```python
from build123d import *

# Parameters (mm, degrees)
F0_R        = 3.175
F1_DEPTH    = 6.35
F2_R        = 3.175
F3_DEPTH    = 6.351
F5_DEPTH    = 6.351
F6_T1_DEPTH = 6.35
F7_R        = 1.5875


# Not quite as in the source:
# - a fillet or chamfer that OpenCascade refuses, or shapes differently, is made with other operations: its cross-section is extruded or revolved along the edge and cut away or added


with BuildPart() as f1:
    # F0 (on Front) → F1 (new body)
    with BuildSketch(Plane.XZ):
        with BuildLine():
            ThreePointArc((32.9955678842, -27.305), (40.1446075924, -23.1775), (40.1446075924, -14.9225))
            Line((40.1446075924, -14.9225), (7.1490397082, 42.2275))
            ThreePointArc((7.1490397082, 42.2275), (0, 46.355), (-7.1490397082, 42.2275))
            Line((-7.1490397082, 42.2275), (-40.1446075924, -14.9225))
            ThreePointArc((-40.1446075924, -14.9225), (-40.1446075924, -23.1775), (-32.9955678842, -27.305))
            Line((-32.9955678842, -27.305), (32.9955678842, -27.305))
        make_face()
        with Locations((-32.9955678842, -19.05)):
            Circle(F0_R, mode=Mode.SUBTRACT)
        with Locations((32.9955678842, -19.05)):
            Circle(F0_R, mode=Mode.SUBTRACT)
        with Locations((0, 38.1)):
            Circle(F0_R, mode=Mode.SUBTRACT)
    extrude(amount=F1_DEPTH)

    # F2 (on face) → F3 (cut, through all)
    with BuildSketch(Plane.XZ.offset(6.35)):
        Circle(F2_R)
    extrude(amount=-F3_DEPTH, mode=Mode.SUBTRACT)

    # F4 (on face) → F5 (cut, through all)
    with BuildSketch(Plane.XZ.offset(6.35)):
        with BuildLine():
            ThreePointArc((-8.255, 0), (-7.1490397082, 4.1275), (-4.1275, 7.1490397082))
            Line((-4.1275, 7.1490397082), (-4.1275, 30.9509602918))
            Line((-4.1275, 30.9509602918), (-28.8680678842, -11.9009602918))
            Line((-28.8680678842, -11.9009602918), (-8.255, 0))
        make_face()
        with BuildLine():
            Line((24.7405678842, -19.05), (4.1275, -7.1490397082))
            ThreePointArc((4.1275, -7.1490397082), (0, -8.255), (-4.1275, -7.1490397082))
            Line((-4.1275, -7.1490397082), (-24.7405678842, -19.05))
            Line((-24.7405678842, -19.05), (24.7405678842, -19.05))
        make_face()
        with BuildLine():
            ThreePointArc((4.1275, 7.1490397082), (7.1490397082, 4.1275), (8.255, 0))
            Line((8.255, 0), (28.8680678842, -11.9009602918))
            Line((28.8680678842, -11.9009602918), (4.1275, 30.9509602918))
            Line((4.1275, 30.9509602918), (4.1275, 7.1490397082))
        make_face()
    extrude(amount=-F5_DEPTH, mode=Mode.SUBTRACT)

    # F6: fillet of radius 25.4 on 6 edges, made by hand

    # F6_s2 → F6_t1 (join)
    with BuildSketch(Plane.XZ):
        with BuildLine():
            ThreePointArc((-7.2425943396, 3.9610418114), (-4.9185930375, 9.8590537015), (-4.1275, 16.1488627696))
            Line((-4.1275, 16.1488627696), (-4.1275, 7.1490397082))
            ThreePointArc((-4.1275, 7.1490397082), (-5.9042860678, 5.7692660737), (-7.2425943396, 3.9610418114))
        make_face()
        with BuildLine():
            ThreePointArc((-16.0490754007, -4.4999115307), (-10.9974874815, -0.6699003293), (-7.0516600039, 4.2917497817))
            ThreePointArc((-7.0516600039, 4.2917497817), (-7.9484740149, 2.2286286891), (-8.255, 0))
            Line((-8.255, 0), (-16.0490754007, -4.4999115307))
        make_face()
        with BuildLine():
            ThreePointArc((0.1909343357, -8.2527915931), (-6.078894444, -9.1891533721), (-11.9215754007, -11.6489512389))
            Line((-11.9215754007, -11.6489512389), (-4.1275, -7.1490397082))
            ThreePointArc((-4.1275, -7.1490397082), (-2.0441879471, -7.9978947628), (0.1909343357, -8.2527915931))
        make_face()
        with BuildLine():
            ThreePointArc((11.9215754007, -11.6489512389), (6.078894444, -9.1891533721), (-0.1909343357, -8.2527915931))
            ThreePointArc((-0.1909343357, -8.2527915931), (2.0441879471, -7.9978947628), (4.1275, -7.1490397082))
            Line((4.1275, -7.1490397082), (11.9215754007, -11.6489512389))
        make_face()
        with BuildLine():
            ThreePointArc((7.0516600039, 4.2917497817), (10.9974874815, -0.6699003293), (16.0490754007, -4.4999115307))
            Line((16.0490754007, -4.4999115307), (8.255, 0))
            ThreePointArc((8.255, 0), (7.9484740149, 2.2286286891), (7.0516600039, 4.2917497817))
        make_face()
        with BuildLine():
            ThreePointArc((4.1275, 16.1488627696), (4.9185930375, 9.8590537015), (7.2425943396, 3.9610418114))
            ThreePointArc((7.2425943396, 3.9610418114), (5.9042860678, 5.7692660737), (4.1275, 7.1490397082))
            Line((4.1275, 7.1490397082), (4.1275, 16.1488627696))
        make_face()
    extrude(amount=F6_T1_DEPTH)

    # F7
    f7_edges = [f1.edges().sort_by_distance(p)[0] for p in [
        (4.1275, -3.175, 30.95096),
        (-4.1275, -3.175, 30.95096),
        (-28.868068, -3.175, -11.90096),
        (28.868068, -3.175, -11.90096),
        (24.740568, -3.175, -19.05),
        (-24.740568, -3.175, -19.05),
    ]]
    fillet(f7_edges, radius=F7_R)


solid = f1.part
```
Work out the finished part from the listing and answer in its coordinate system (mm). A direction names the side the tool comes from. Round coordinates to 2 decimals unless told otherwise and drop trailing zeros. Order: outer loops, then holes, each group sorted by start corner. A loop starts at its lowest first (then second) coordinate and runs counter-clockwise, first axis right, second up.
Q1. A cutting plane is placed at B-B, the plane z = 10. Determine the outline of the cut face in (x, y).
Solution:
outline: (-25.76, -6.35) - (-16.22, -6.35) - (-16.22, 0) - (-25.76, 0) - close; (-4.88, -6.35) - (4.88, -6.35) - (4.88, 0) - (-4.88, 0) - close; (16.22, -6.35) - (25.76, -6.35) - (25.76, 0) - (16.22, 0) - close
Q2. A cutting plane is placed at C-C, the plane x = -8.5. Determine the outline of the cut face in (y, z) (3 decimals).
Solution:
outline: (-6.35, -27.305) - (0, -27.305) - (0, -19.05) - (-6.35, -19.05) - close; (-6.35, -10.001) - (0, -10.001) - (0, 2.163) - (-6.35, 2.163) - close; (-6.35, 23.378) - (0, 23.378) - (0, 39.888) - (-6.35, 39.888) - close
Q3. The mould has two halves that part along Z. Classify faces 3 (the flat face through (0, -3, -27.305)), 4 (the flat face through (-15.712, -3.219, -13.837)), 5 (the cylindrical face through (40.083, -3.131, -23.282)): pulls with the +Z half, pulls with the -Z half, needs draft (parallel to the pull), parting line crosses it, or undercut.
Solution:
face 3: pulls with the -Z half
face 4: undercut
face 5: parting line crosses it
Q4. A cutting plane is placed at D-D, the plane z = 0. Determine the outline of the cut face in (x, y) (3 decimals).
Solution:
outline: (-31.529, -6.35) - (-21.997, -6.35) - (-21.997, 0) - (-31.529, 0) - close; (-10.337, -6.35) - (-3.175, -6.35) - (-3.175, 0) - (-10.337, 0) - close; (3.175, -6.35) - (10.337, -6.35) - (10.337, 0) - (3.175, 0) - close; (21.997, -6.35) - (31.529, -6.35) - (31.529, 0) - (21.997, 0) - close
Q5. Find the intervals of material crossed by line 1 along Z through (x, y) = (-6, -4.5) (3 decimals); line 2 along X through (y, z) = (-2.5, 10.5); line 3 along Z through (x, y) = (12, -1.5) (3 decimals), in increasing order.
Solution:
line 1: z = -27.305 to -19.05, -9.167 to 6.577, 26.588 to 43.77
line 2: x = -25.47 to -15.93, -4.76 to 4.76, 15.93 to 25.47
line 3: z = -27.305 to -19.05, -11.694 to -1.598, 17.315 to 33.825
Q6. A tool of negligible diameter and unlimited length cuts with its end or side. For faces 1 (the flat face through (-19.95, -3.22, -6.75)), 2 (the flat face through (23.88, -3.13, 13.25)), from which of +Z, -Z, +X, -X, +Y, -Y can it reach the whole face along a straight path? Write none if from no direction.
Solution:
face 1: +Y, -Y
face 2: +Z, +X, +Y, -Y
Q7. Given pin 1 Ø3 at (y, z) = (-2, 34.5) entering from +X; pin 2 Ø6 at (x, z) = (-18, 33) entering from +Y (1 decimal); pin 3 Ø2 at (x, y) = (-3.5, -5) entering from +Z, each flat-ended and moving along its own axis, determine where each tip first touches the part or whether it passes through.
Solution:
pin 1: stops at x = 12.48
pin 2: passes through
pin 3: stops at z = 45.97
Q8. A cutting plane is placed at A-A, the plane y = -1.75. Count the separate pieces of the cut face and the enclosed holes in it, then the cut area to 3 significant figures.
Solution:
separate pieces: 1
enclosed holes: 7
area: 2,670 mm2
